Read the model definition and answer for the solid it produces. Units are mm, in the model's axes. Face numbers are marked on the shaded views. A direction names the side the tool comes from. Give positions to 0.01 mm unless a question says otherwise; leave off trailing zeros. Loops run counter-clockwise (first coordinate to the right, second up) from the corner with the lowest first, then second, coordinate; pieces in that order, holes last.
(1) Which of the six approach directions +Z, -Z, +X, -X, +Y, -Y give full straight-line access (tool end or side, diameter ignored) to the marked faces 1 and 2?
(2) This flat-tipped pin is pushed along its axis until it touches: P1, Ø1.5, axis at y = 9.5, z = 2, coming from the +X side. Where does it stop, or does it pass through?
(3) Find section A-A, the plane y = -2. Write down the section's boundary in (x, z), then the cut area to 3 significant figures.
(4) Straight lines are drawn through the part: probe 1 along X at (y, z) = (6, 1); probe 2 along Y at (x, z) = (-6, 0.85); probe 3 along Y at (x, z) = (5.75, 1.55). For each, find the intervals that lie inside material, in ascending order.
(5) Find section D-D, the plane y = -11. Write down the section's boundary in (x, z), then the cut area to 3 significant figures.
(6) Determine the mould class of the marked faces 3, 4 and 5 for opening direction Y: pulls with the +Y half, pulls with the -Y half, needs draft (parallel to the pull), parting line crosses it, or undercut.
(7) Find section B-B, the plane x = 8.5. Write down the section's boundary in (y, z).
(8) Find section C-C, the plane z = 2.15. Write down the section's boundary in (x, y), then the cut area to 3 significant figures.
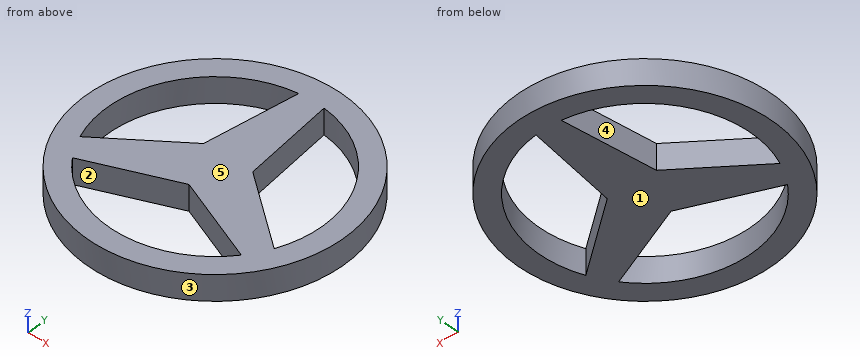
```python
from build123d import *

# Parameters (mm, degrees)
SKETCH_1_R      = 15
SKETCH_1_R_2    = 12.5
EXTRUDE_1_DEPTH = 3


with BuildPart() as part:
    # 草图1 → 凸台-拉伸1 (new body)
    # profile 1 of 2: a face of its own
    with BuildSketch(Plane.XY):
        Circle(SKETCH_1_R)
        Circle(SKETCH_1_R_2, mode=Mode.SUBTRACT)
    # profile 2 of 2: a face of its own
    with BuildSketch(Plane.XY):
        with BuildLine():
            ThreePointArc((1.5, 12.409673646), (0, 12.5), (-1.5, 12.409673646))
            Line((-1.5, 12.409673646), (-2.912394569, 1.681471788))
            Line((-2.912394569, 1.681471788), (-11.49709263, -4.905798717))
            ThreePointArc((-11.49709263, -4.905798717), (-10.825317547, -6.25), (-9.99709263, -7.503874929))
            Line((-9.99709263, -7.503874929), (0, -3.362943577))
            Line((0, -3.362943577), (9.99709263, -7.503874929))
            ThreePointArc((9.99709263, -7.503874929), (10.825317547, -6.25), (11.49709263, -4.905798717))
            Line((11.49709263, -4.905798717), (2.912394569, 1.681471788))
            Line((2.912394569, 1.681471788), (1.5, 12.409673646))
        make_face()
    extrude(amount=EXTRUDE_1_DEPTH)


solid = part.part
```
Entries:
1. face 1: -Z, +X, -X, +Y, -Y
1. face 2: +Z, -Z
2. P1: stops at x = 12.18
3. outline: (-14.87, 0) - (-12.34, 0) - (-12.34, 3) - (-14.87, 3) - close; (-7.71, 0) - (7.71, 0) - (7.71, 3) - (-7.71, 3) - close; (12.34, 0) - (14.87, 0) - (14.87, 3) - (12.34, 3) - close
3. area: 61.4 mm2
4. probe 1: x = -13.75 to -10.97, -2.34 to 2.34, 10.97 to 13.75
4. probe 2: y = -13.75 to -10.97, -5.85 to -0.69, 10.97 to 13.75
4. probe 3: y = -13.85 to -11.1, -5.74 to -0.5, 11.1 to 13.85
5. outline: (-10.2, 0) - (-5.94, 0) - (-5.94, 3) - (-10.2, 3) - close; (5.94, 0) - (10.2, 0) - (10.2, 3) - (5.94, 3) - close
5. area: 25.6 mm2
6. face 3: parting line crosses it
6. face 4: undercut
6. face 5: needs draft
7. outline: (-12.36, 0) - (-9.17, 0) - (-9.17, 3) - (-12.36, 3) - close; (-6.88, 0) - (-2.61, 0) - (-2.61, 3) - (-6.88, 3) - close; (9.17, 0) - (12.36, 0) - (12.36, 3) - (9.17, 3) - close
8. outline: circle Ø30 at (0, 0); hole (-11.5, -4.91) - (-2.91, 1.68) - (-1.5, 12.41) arc R12.5 ccw to start; hole (-10, -7.5) arc R12.5 ccw to (10, -7.5) - (0, -3.36) - close; hole (1.5, 12.41) - (2.91, 1.68) - (11.5, -4.91) arc R12.5 ccw to start
8. area: 373 mm2
